Part print with two shaded views. Sizes in mm from the minimum x, y, z corner. Give positions to 0.01 mm unless a question says otherwise; leave off trailing zeros. Write each loop counter-clockwise with the first axis right and the second up, starting at its lowest first coordinate (ties: lowest second). Pieces come first, ordered by that corner, then holes.
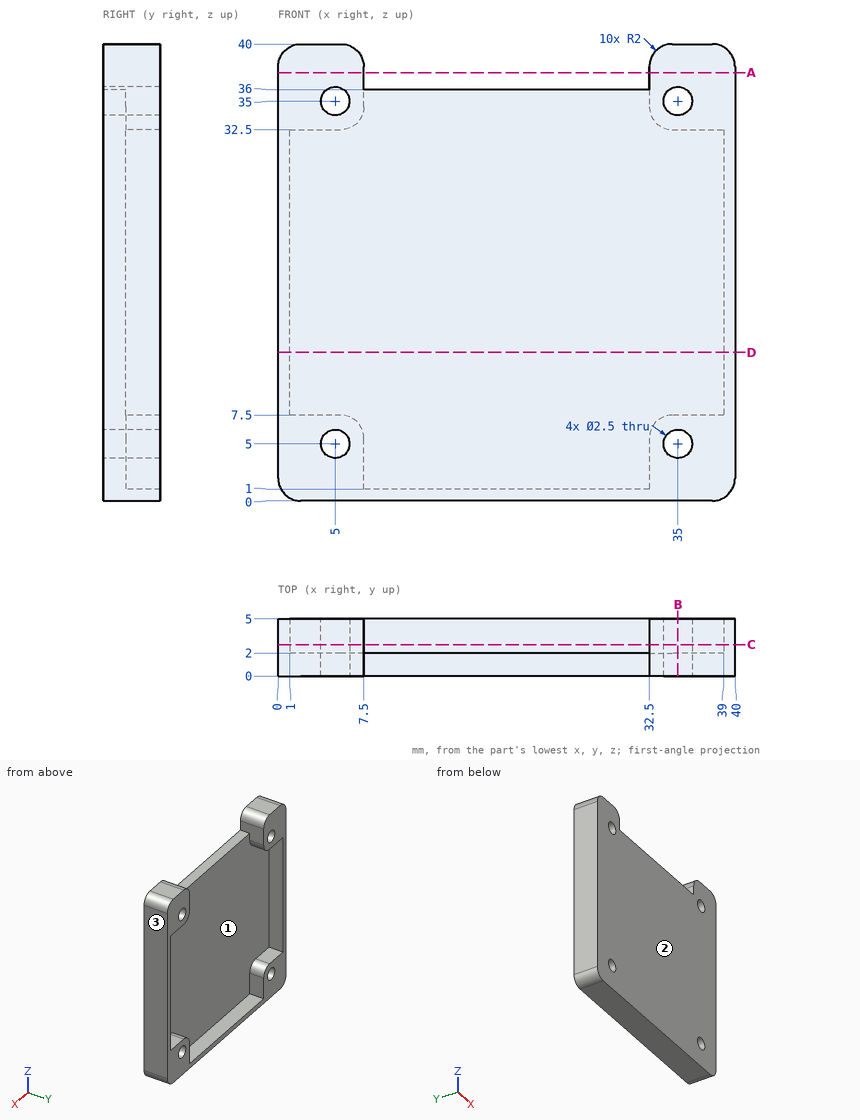
1) Two-plate mould, pull along X, no slides. Class the marked faces 1, 2 and 3: +X half, -X half, draft (parallel to the pull), parting line (faces both ways), or undercut.
Answers follow:
face 1: undercut
face 2: draft
face 3: +X half
2) Saw through at C-C, the plane y = 2.75. Count the separate pieces of the cut face and the enclosed holes in it, then the cut area to 3 significant figures.
Answers follow:
separate pieces: 1
enclosed holes: 4
area: 272 mm2
3) Saw through at D-D, the plane z = 13. Write the cut outline in (x, y).
Answers follow:
outline: (0, 0) - (40, 0) - (40, 5) - (39, 5) - (39, 2) - (1, 2) - (1, 5) - (0, 5) - close
4) Saw through at A-A, the plane z = 37.5. Write the cut outline in (x, y).
Answers follow:
outline: (0, 0) - (7.5, 0) - (7.5, 5) - (0, 5) - close; (32.5, 0) - (40, 0) - (40, 5) - (32.5, 5) - close
5) Wall check: L1, parallel to Z at x = 35, y = 2.7; L2, parallel to X at y = 0.6, z = 37; L3, parallel to X at y = 2.35, z = 36. Give the ranges that are in metal, low to high.
Answers follow:
L1: z = 0 to 3.75, 6.25 to 7.5, 32.5 to 33.75, 36.25 to 40
L2: x = 0 to 7.5, 32.5 to 40
L3: x = 0 to 4.25, 5.75 to 7.5, 32.5 to 34.25, 35.75 to 40
6) Pin check, flat tips, straight feed: pin 1 Ø0.6 at (x, y) = (26, 1.5) entering from +Z; pin 2 Ø10.5 at (x, z) = (12.5, 21) entering from +Y; pin 3 Ø2 at (x, y) = (20.5, 3.5) entering from +Z. Stop position of each tip, or through.
Answers follow:
pin 1: stops at z = 36
pin 2: stops at y = 2
pin 3: stops at z = 1
7) Saw through at B-B, the plane x = 35. Write the cut outline in (y, z), then the cut area to 3 significant figures.
Answers follow:
outline: (0, 0) - (5, 0) - (5, 3.75) - (0, 3.75) - close; (0, 6.25) - (5, 6.25) - (5, 7.5) - (2, 7.5) - (2, 32.5) - (5, 32.5) - (5, 33.75) - (0, 33.75) - close; (0, 36.25) - (5, 36.25) - (5, 40) - (0, 40) - close
area: 100 mm2
